Input: part model. Units: mm. Frame: model coordinates. Face numbers are marked on the shaded views. A direction names the side the tool comes from. Round coordinates to 2 decimals unless told otherwise and drop trailing zeros. Write each loop counter-clockwise with the first axis right and the second up, starting at its lowest first coordinate (ties: lowest second). Pieces come first, ordered by that corner, then holes. Notation, with made-up numbers: M 65.25,13 L 113.25,13 A6 cw 113.25,18 Z; hole C 55.25,77.5 d1. An arc over 180 degrees is marked long. Use one line per item in the form item = value. Start each with the question number.
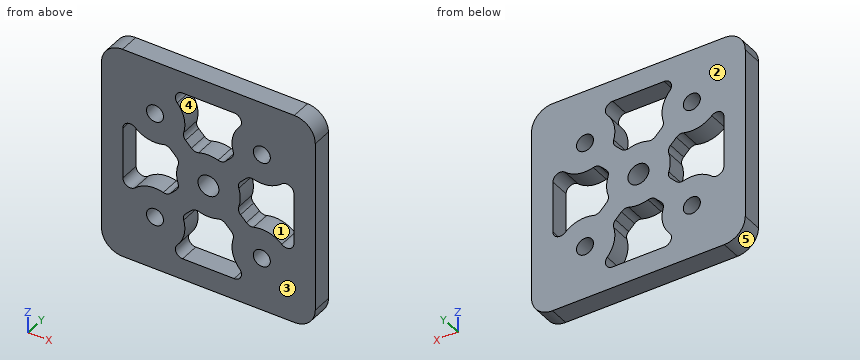
Autodesk Inventor part; units mm, degrees
ref_plane "YZ Plane" through (0, 0, 0) normal (1, 0, 0) x (0, 1, 0)
ref_plane "XZ Plane" through (0, 0, 0) normal (0, 1, 0) x (-1, 0, 0)
ref_plane "XY Plane" through (0, 0, 0) normal (0, 0, 1) x (1, 0, 0)
sketch "Sketch2" plane through (0, 0, 0) normal (0, 1, 0) x (-1, 0, 0)
  line L0 (45.8216, 45.8216) -> (4.9784, 45.8216)
  arc A0 (4.9784, 45.8216) -> (0, 40.8432) centre (4.9784, 40.8432) ccw
  line L1 (0, 40.8432) -> (0, 0)
  arc A1 (0, 0) -> (4.9784, -4.9784) centre (4.9784, 0) ccw
  line L2 (4.9784, -4.9784) -> (45.8216, -4.9784)
  arc A2 (45.8216, -4.9784) -> (50.8, 0) centre (45.8216, 0) ccw
  line L3 (50.8, 0) -> (50.8, 40.8432)
  arc A3 (50.8, 40.8432) -> (45.8216, 45.8216) centre (45.8216, 40.8432) ccw
  arc A4 (33.0362, 24.4657) -> (32.6118, 22.7199) centre (34.2575, 23.2444) ccw
  line L4 (33.0362, 24.4657) -> (34.4326, 25.8621)
  arc A5 (36.1326, 26.3004) -> (34.4326, 25.8621) centre (35.6539, 24.6408) ccw
  arc A6 (36.1326, 26.3004) -> (42.8397, 27.8362) centre (38.1, 33.1216) ccw
  arc A7 (45.72, 26.5503) -> (42.8397, 27.8362) centre (43.9928, 26.5503) ccw
  line L5 (45.72, 26.5503) -> (45.72, 14.2929)
  arc A8 (42.8397, 13.007) -> (45.72, 14.2929) centre (43.9928, 14.2929) ccw
  arc A9 (42.8397, 13.007) -> (36.1326, 14.5428) centre (38.1, 7.7216) ccw
  arc A10 (34.4326, 14.9811) -> (36.1326, 14.5428) centre (35.6539, 16.2024) ccw
  line L6 (34.4326, 14.9811) -> (33.0362, 16.3775)
  arc A11 (32.6118, 18.1233) -> (33.0362, 16.3775) centre (34.2575, 17.5988) ccw
  arc A12 (32.6118, 18.1233) -> (32.6118, 22.7199) centre (25.4, 20.4216) ccw
  arc A13 (17.7638, 16.3775) -> (18.1882, 18.1233) centre (16.5425, 17.5988) ccw
  line L7 (17.7638, 16.3775) -> (16.3674, 14.9811)
  arc A14 (14.6674, 14.5428) -> (16.3674, 14.9811) centre (15.1461, 16.2024) ccw
  arc A15 (14.6674, 14.5428) -> (7.9603, 13.007) centre (12.7, 7.7216) ccw
  arc A16 (5.08, 14.2929) -> (7.9603, 13.007) centre (6.8072, 14.2929) ccw
  line L8 (5.08, 14.2929) -> (5.08, 26.5503)
  arc A17 (7.9603, 27.8362) -> (5.08, 26.5503) centre (6.8072, 26.5503) ccw
  arc A18 (7.9603, 27.8362) -> (14.6674, 26.3004) centre (12.7, 33.1216) ccw
  arc A19 (16.3674, 25.8621) -> (14.6674, 26.3004) centre (15.1461, 24.6408) ccw
  line L9 (16.3674, 25.8621) -> (17.7638, 24.4657)
  arc A20 (18.1882, 22.7199) -> (17.7638, 24.4657) centre (16.5425, 23.2444) ccw
  arc A21 (18.1882, 22.7199) -> (18.1882, 18.1233) centre (25.4, 20.4216) ccw
  arc A22 (30.8405, 29.4542) -> (31.2788, 31.1542) centre (29.6192, 30.6755) ccw
  line L10 (30.8405, 29.4542) -> (29.4441, 28.0578)
  arc A23 (27.6983, 27.6334) -> (29.4441, 28.0578) centre (28.2228, 29.2791) ccw
  arc A24 (27.6983, 27.6334) -> (23.1017, 27.6334) centre (25.4, 20.4216) ccw
  arc A25 (21.3559, 28.0578) -> (23.1017, 27.6334) centre (22.5772, 29.2791) ccw
  line L11 (21.3559, 28.0578) -> (19.9595, 29.4542)
  arc A26 (19.5212, 31.1542) -> (19.9595, 29.4542) centre (21.1808, 30.6755) ccw
  arc A27 (19.5212, 31.1542) -> (17.9854, 37.8613) centre (12.7, 33.1216) ccw
  arc A28 (19.2713, 40.7416) -> (17.9854, 37.8613) centre (19.2713, 39.0144) ccw
  line L12 (19.2713, 40.7416) -> (31.5287, 40.7416)
  arc A29 (32.8146, 37.8613) -> (31.5287, 40.7416) centre (31.5287, 39.0144) ccw
  arc A30 (32.8146, 37.8613) -> (31.2788, 31.1542) centre (38.1, 33.1216) ccw
  arc A31 (19.9595, 11.389) -> (19.5212, 9.689) centre (21.1808, 10.1677) ccw
  line L13 (19.9595, 11.389) -> (21.3559, 12.7854)
  arc A32 (23.1017, 13.2098) -> (21.3559, 12.7854) centre (22.5772, 11.5641) ccw
  arc A33 (23.1017, 13.2098) -> (27.6983, 13.2098) centre (25.4, 20.4216) ccw
  arc A34 (29.4441, 12.7854) -> (27.6983, 13.2098) centre (28.2228, 11.5641) ccw
  line L14 (29.4441, 12.7854) -> (30.8405, 11.389)
  arc A35 (31.2788, 9.689) -> (30.8405, 11.389) centre (29.6192, 10.1677) ccw
  arc A36 (31.2788, 9.689) -> (32.8146, 2.9819) centre (38.1, 7.7216) ccw
  arc A37 (31.5287, 0.1016) -> (32.8146, 2.9819) centre (31.5287, 1.8288) ccw
  line L15 (31.5287, 0.1016) -> (19.2713, 0.1016)
  arc A38 (17.9854, 2.9819) -> (19.2713, 0.1016) centre (19.2713, 1.8288) ccw
  arc A39 (17.9854, 2.9819) -> (19.5212, 9.689) centre (12.7, 7.7216) ccw
  circle A40 centre (12.7, 7.7216) radius 2.0193
  circle A41 centre (12.7, 33.1216) radius 2.0193
  circle A42 centre (38.1, 33.1216) radius 2.0193
  circle A43 centre (38.1, 7.7216) radius 2.0193
  circle A44 centre (25.4, 20.4216) radius 2.4892
  point P0 (0, 40.8432)
  point P1 (4.9784, -4.9784)
  point P2 (50.8, 0)
  point P3 (23.1017, 13.2098)
  point P4 (27.6983, 13.2098)
  point P5 (29.4441, 12.7854)
  point P6 (32.8146, 2.9819)
  point P7 (31.5287, 0.1016)
  point P8 (17.9854, 2.9819)
  point P9 (19.5212, 9.689)
  point P10 (19.5212, 31.1542)
  point P11 (7.9603, 13.007)
  point P12 (5.08, 14.2929)
  point P13 (7.9603, 27.8362)
  point P14 (14.6674, 26.3004)
  point P15 (36.1326, 26.3004)
  point P16 (42.8397, 13.007)
  point P17 (36.1326, 14.5428)
  point P18 (34.4326, 14.9811)
extrude "Plate2" add sketch "Sketch2" along normal blind 4.7625
equation "\"d11\" = Thickness"
equation "\"BendRadius\" = 1.5 * Thickness"
equation "\"BendReliefWidth\" = Thickness"
equation "\"BendReliefDepth\" = 0.5 * Thickness"
equation "\"CornerReliefSize\" = 4 * Thickness"
equation "\"MinimumRemnant\" = 2 * Thickness"
equation "\"TransitionRadius\" = BendRadius"
equation "\"JacobiRadiusSize\" = BendRadius"
equation "\"GapSize\" = Thickness"
properties part number "climber-axle-endcap" material "Polycarbonate, Clear"
Item 1: Cut plane A-A (x = -25.4). Output: boundary loops of the cut face in (y, z), plus the area to 3 significant figures.
Item 2: Cut plane C-C (y = 1.4). Give the number of separate pieces and of enclosed holes in the cut face, plus the area to 3 significant figures.
Item 3: Reachability of the marked faces 1 and 2 from +Z, -Z, +X, -X, +Y, -Y: full face, straight path, thin tool, end or side. Return the list, or none.
Item 4: Cut plane B-B (z = 9). Output: boundary loops of the cut face in (x, y).
Item 5: Draft query along Z for the marked faces 3, 4 and 5. Return one class per face: +Z half, -Z half, draft (parallel to the pull), parting line (faces both ways), or undercut.
Item 6: Ray query, line 1 (Z direction, x = -25.4, y = 2.8); line 2 (Z direction, x = -38.1, y = 1.5); line 3 (Z direction, x = -28.5, y = 1.45). Return the intervals inside material, ascending. Write a range as from..to.
Final values:
q1.outline = M 0,-4.98 L 4.76,-4.98 L 4.76,0.1 L 0,0.1 Z; M 0,12.85 L 4.76,12.85 L 4.76,17.93 L 0,17.93 Z; M 0,22.91 L 4.76,22.91 L 4.76,27.99 L 0,27.99 Z; M 0,40.74 L 4.76,40.74 L 4.76,45.82 L 0,45.82 Z
q1.area = 96.8 mm^2
q2.separate_pieces = 1
q2.enclosed_holes = 9
q2.area = 1,850 mm^2
q3.face_1 = +Y, -Y
q3.face_2 = +Z, -Z, +X, -X, +Y
q4.outline = M -50.8,0 L -39.66,0 L -39.66,4.76 L -50.8,4.76 Z; M -36.54,0 L -31.12,0 L -31.12,4.76 L -36.54,4.76 Z; M -19.68,0 L -14.26,0 L -14.26,4.76 L -19.68,4.76 Z; M -11.14,0 L 0,0 L 0,4.76 L -11.14,4.76 Z
q5.face_3 = draft
q5.face_4 = undercut
q5.face_5 = -Z half
q6.line_1 = -4.98..0.1, 12.85..17.93, 22.91..27.99, 40.74..45.82
q6.line_2 = -4.98..5.7, 9.74..14.82, 26.02..31.1, 35.14..45.82
q6.line_3 = -4.98..0.1, 13.27..27.57, 40.74..45.82
